Job drawing, mm, ordinate dimensions from the low corner. One solid piece. A direction names the side the tool comes from. Give positions to 0.01 mm unless a question says otherwise; leave off trailing zeros. Write each loop counter-clockwise with the first axis right and the second up, starting at its lowest first coordinate (ties: lowest second). Pieces come first, ordered by that corner, then holes. Notation, with made-up numbers: (79.25, -19) - (102.25, -19) arc R27 cw to (102.25, -3) - close; hole circle Ø6 at (51.25, -17). An arc over 180 degrees is marked (long way). Answer in a Markdown table with one row per item. Add a question column.
1. Which spindle directions (+Z, -Z, +X, -X, +Y, -Y) get a long thin tool onto all of the face, cutting with end or side? Do the marked faces 1 and 2. Say none if no direction does.
2. Band-saw the part on C-C on x = 33.5. Write the cut outline in (y, z), plus the area to 3 significant figures.
3. Band-saw the part on B-B on y = 11. Write the cut outline in (x, z), plus the area to 3 significant figures.
4. Band-saw the part on A-A on z = 24.5. Write the cut outline in (x, y) (1 decimal).
5. Band-saw the part on D-D on z = 29. Write the cut outline in (x, y) (1 decimal).
6. Probe line 1 along X through (y, z) = (19, 19.5); line 2 along Y through (x, z) = (58.35, 2.4) (1 decimal); line 3 along Z through (x, y) = (24.5, 25). List the from-to ranges inside material, lowest first.
7. Drop flat-ended pins along their axis: pin 1 Ø10 at (x, z) = (7, 15.5) entering from +Y; pin 2 Ø2 at (x, z) = (2.5, 33.5) entering from +Y; pin 3 Ø0.8 at (y, z) = (33.5, 34) entering from +X; pin 4 Ø2.5 at (y, z) = (15.07, 2.4) entering from +X. Give the stop position or say it passes through.
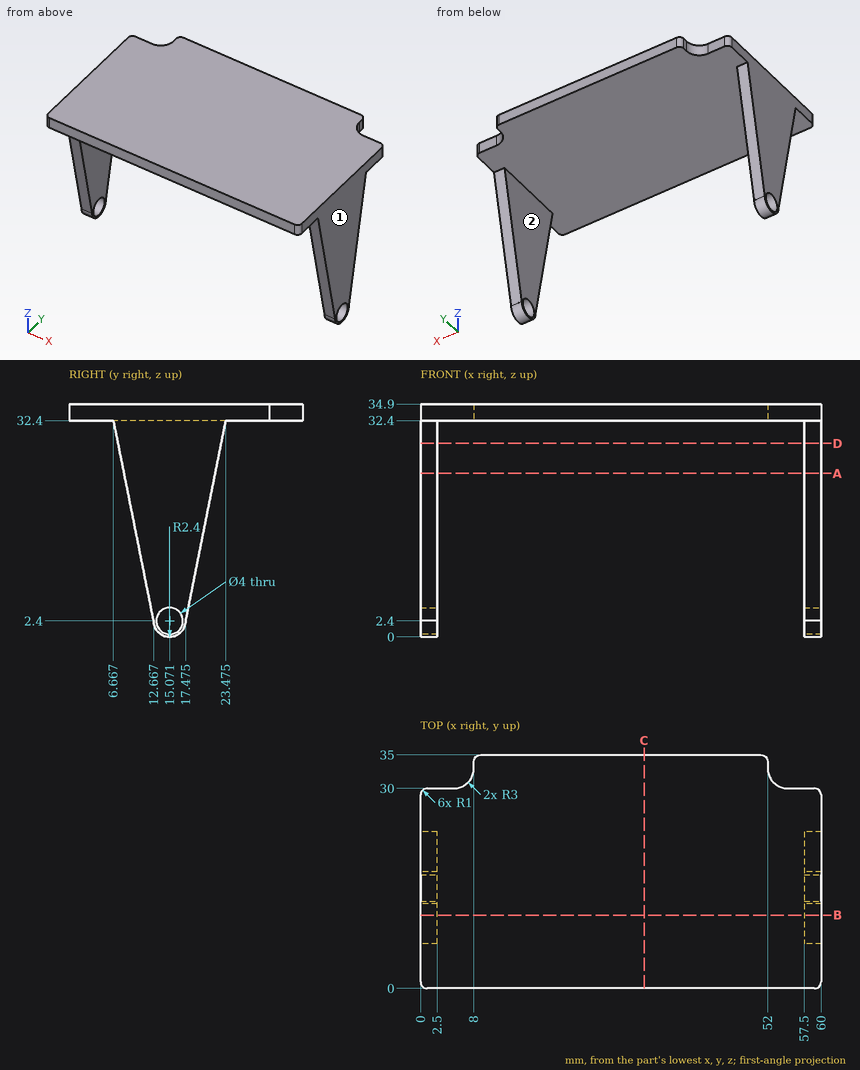
Values:
| question | item | result |
|---|---|---|
| 1 | face 1 | +Z, -Z, +X, +Y, -Y |
| 1 | face 2 | -Z, +Y, -Y |
| 2 | outline | (0, 32.4) - (35, 32.4) - (35, 34.9) - (0, 34.9) - close |
| 2 | area | 87.5 mm² |
| 3 | outline | (0, 10.74) - (2.5, 10.74) - (2.5, 32.4) - (57.5, 32.4) - (57.5, 10.74) - (60, 10.74) - (60, 34.9) - (0, 34.9) - close |
| 3 | area | 258 mm² |
| 4 | outline | (0, 8.2) - (2.5, 8.2) - (2.5, 21.9) - (0, 21.9) - close; (57.5, 8.2) - (60, 8.2) - (60, 21.9) - (57.5, 21.9) - close |
| 5 | outline | (0, 7.3) - (2.5, 7.3) - (2.5, 22.8) - (0, 22.8) - close; (57.5, 7.3) - (60, 7.3) - (60, 22.8) - (57.5, 22.8) - close |
| 6 | line 1 | x = 0 to 2.5, 57.5 to 60 |
| 6 | line 2 | y = 12.7 to 13.1, 17.1 to 17.5 |
| 6 | line 3 | z = 32.4 to 34.9 |
| 7 | pin 1 | stops at y = 20.53 |
| 7 | pin 2 | stops at y = 30 |
| 7 | pin 3 | stops at x = 52 |
| 7 | pin 4 | passes through |
